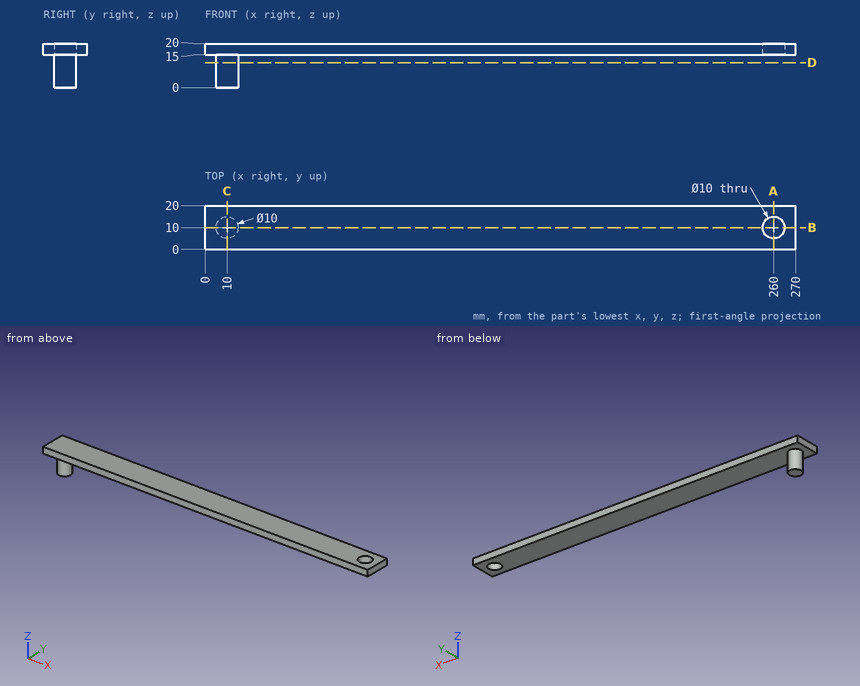
Geometry: see drawing. Coordinates: mm, zero at the bounding-box minimum. Coordinates: 2 decimals unless noted, no trailing zeros. Loops run counter-clockwise (first coordinate to the right, second up) from the corner with the lowest first, then second, coordinate; pieces in that order, holes last. Notation, with made-up numbers: M 2,42.25 L 7,42.25 A30 cw 7,75.25 Z; hole C 19,28 d7. An arc over 180 degrees is marked long. Answer in a Markdown table with one row per item.
Q1. First-contact query: pin 1 (8 mm diameter, centred on x = 218.5, y = 6, fed in from -Z); pin 2 (4 mm diameter, centred on y = 3.5, z = 5.5, fed in from -X). Flat tips, straight axial feed; report the tip coordinate or a pass-through.
Answers below:
| item | result |
|---|---|
| pin 1 | stops at z = 15 |
| pin 2 | stops at x = 7.82 |
Q2. Ray query, probe 1 along Y at (x, z) = (260, 17.55); probe 2 along X at (y, z) = (10.5, 15.75); probe 3 along Z at (x, y) = (69, 2.25). Return the intervals inside material, ascending. Write a range as from..to.
Answers below:
| item | result |
|---|---|
| probe 1 | y = 0..5, 15..20 |
| probe 2 | x = 0..255.03, 264.97..270 |
| probe 3 | z = 15..20 |
Q3. Section C-C on x = 10. Return the cut outline in (y, z), plus the area to 3 significant figures.
Answers below:
| item | result |
|---|---|
| outline | M 0,15 L 5,15 L 5,0 L 15,0 L 15,15 L 20,15 L 20,20 L 0,20 Z |
| area | 250 mm^2 |
Q4. Section D-D on z = 11.5. Return the cut outline in (x, y), plus the area to 3 significant figures.
Answers below:
| item | result |
|---|---|
| outline | C 10,10 d10 |
| area | 78.5 mm^2 |
Q5. Section B-B on y = 10. Return the cut outline in (x, z).
Answers below:
| item | result |
|---|---|
| outline | M 0,15 L 5,15 L 5,0 L 15,0 L 15,15 L 255,15 L 255,20 L 0,20 Z; M 265,15 L 270,15 L 270,20 L 265,20 Z |
Q6. Section A-A on x = 260. Return the cut outline in (y, z), plus the area to 3 significant figures.
Answers below:
| item | result |
|---|---|
| outline | M 0,15 L 5,15 L 5,20 L 0,20 Z; M 15,15 L 20,15 L 20,20 L 15,20 Z |
| area | 50.0 mm^2 |
